Geometry check sheet. Reference: drawing and pictorial views, mm from the part's lowest x, y, z. A direction names the side the tool comes from. Round coordinates to 2 decimals unless told otherwise and drop trailing zeros. Loops run counter-clockwise (first coordinate to the right, second up) from the corner with the lowest first, then second, coordinate; pieces in that order, holes last. Notation, with made-up numbers: (-40, -20) - (-27, -20) arc R25 cw to (-27, 7) - close; hole circle Ø2 at (18.25, 64.25). An arc over 180 degrees is marked (long way). Return JSON: item names as keys, results as strings.
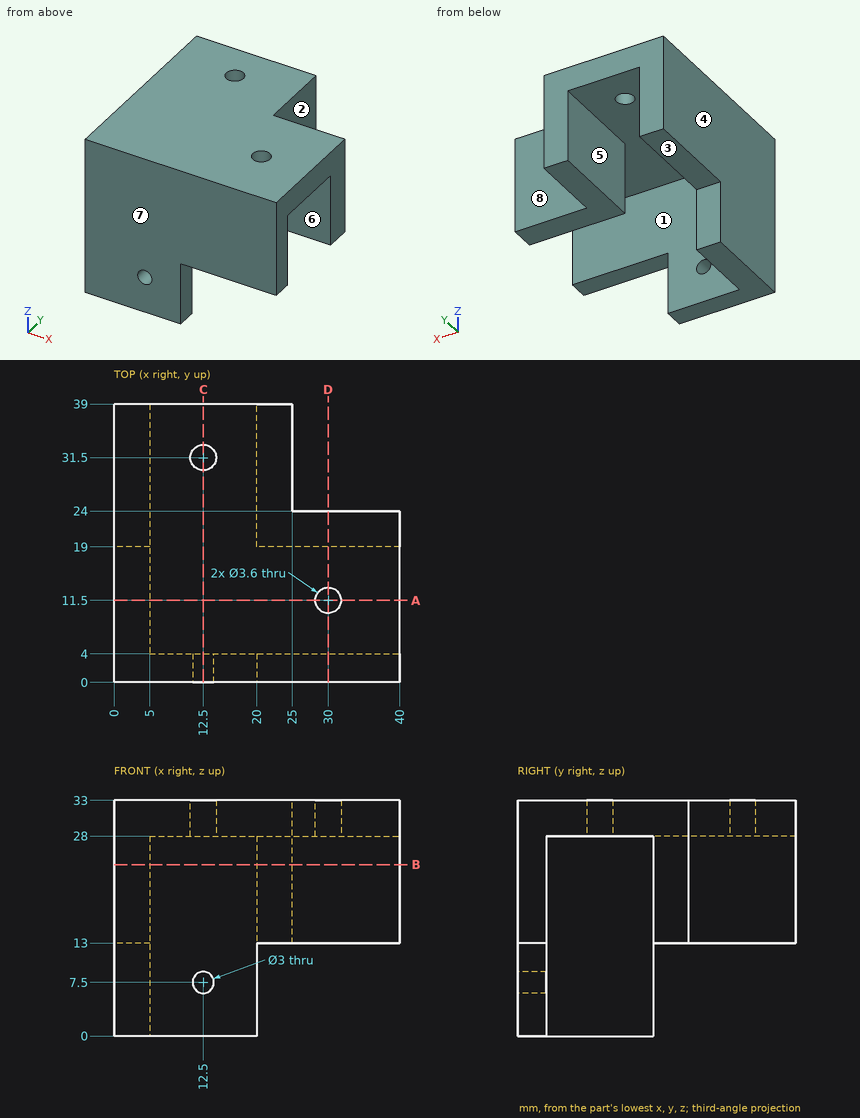
Q1. Sectioned sample at A-A (y = 11.5). Enter the section's corners in (x, z).
Answer key:
{"outline": "(0, 0) - (5, 0) - (5, 28) - (28.2, 28) - (28.2, 33) - (0, 33) - close; (31.8, 28) - (40, 28) - (40, 33) - (31.8, 33) - close"}
Q2. Draft check along Y on the marked faces 5, 6, 7 and 8. Enter one of: released by +Y, released by -Y, zero draft, split by the parting line, or undercut.
Answer key:
{"face 5": "zero draft", "face 6": "undercut", "face 7": "released by -Y", "face 8": "released by +Y"}
Q3. Depth check by flat-ended pin: P1, Ø5.5, axis at x = 3, z = 7, coming from the +Y side; P2, Ø4.5, axis at y = 1, z = 6, coming from the +X side; P3, Ø1.5, axis at x = 21, z = 11.5, coming from the -Y side; P4, Ø17.5, axis at x = 28, y = 25, coming from the -Z side. Enter the tip coordinate at first touch or a pass-through.
Answer key:
{"P1": "stops at y = 19", "P2": "stops at x = 20", "P3": "passes through", "P4": "stops at z = 13"}
Q4. Scan lines: probe 1 along X at (y, z) = (28, 17); probe 2 along Y at (x, z) = (38, 16); probe 3 along Z at (x, y) = (19, 31). Record each from-to range of solid material in increasing order. Write a range as [from, to].
Answer key:
{"probe 1": "x = [0, 5], [20, 25]", "probe 2": "y = [0, 4], [19, 24]", "probe 3": "z = [28, 33]"}
Q5. Sectioned sample at D-D (x = 30). Enter the section's corners in (y, z), plus the area to 3 significant figures.
Answer key:
{"outline": "(0, 13) - (4, 13) - (4, 28) - (9.7, 28) - (9.7, 33) - (0, 33) - close; (13.3, 28) - (19, 28) - (19, 13) - (24, 13) - (24, 33) - (13.3, 33) - close", "area": "237 mm²"}
Q6. Sectioned sample at B-B (z = 24). Enter the section's corners in (x, y).
Answer key:
{"outline": "(0, 0) - (40, 0) - (40, 4) - (5, 4) - (5, 39) - (0, 39) - close; (20, 19) - (40, 19) - (40, 24) - (25, 24) - (25, 39) - (20, 39) - close"}
Q7. Tool access check on the marked faces 1, 2, 3 and 4. Record the directions out of +Z, -Z, +X, -X, +Y, -Y that give a thin tool (end or side, any length) a straight path to the whole face; none if there is none.
Answer key:
{"face 1": "-Z, +X", "face 2": "+Z, -Z, +X, +Y", "face 3": "-Z, +X, -X, +Y", "face 4": "+Z, -Z, -X, +Y, -Y"}
Q8. Sectioned sample at C-C (x = 12.5). Enter the section's corners in (y, z).
Answer key:
{"outline": "(0, 0) - (4, 0) - (4, 6) - (0, 6) - close; (0, 9) - (4, 9) - (4, 28) - (29.7, 28) - (29.7, 33) - (0, 33) - close; (33.3, 28) - (39, 28) - (39, 33) - (33.3, 33) - close"}
